Source: CAD feature listing. Evaluate the final solid. Frame: model axes, mm. A direction names the side the tool comes from. Give positions to 0.01 mm unless a question says otherwise; leave off trailing zeros. Order: outer loops, then holes, each group sorted by start corner. A loop starts at its lowest first (then second) coordinate and runs counter-clockwise, first axis right, second up. Notation, with made-up numbers: M -22,39.25 L 2,39.25 A27 ccw 2,63.25 Z; hole C -7.5,-10.5 d9. An arc over 180 degrees is marked long. Answer as a JSON object with one key per item and string values. Group by question number.
1. Section query D-D (x = -15). Output: boundary loops of the cut face in (y, z), plus the area to 3 significant figures.
2. Pin query (flat end, axial travel): P1, Ø8, axis at x = -4, z = 11, coming from the -Y side; P2, Ø3.5, axis at y = -14.5, z = 22, coming from the -X side; P3, Ø8, axis at x = 30, z = -2.5, coming from the -Y side; P4, Ø8, axis at x = 24, y = -16, coming from the +Z side. Return the tip coordinate at first contact, or that it passes through.
3. Material intervals for L1, parallel to Y at x = -6, z = -1; L2, parallel to Y at x = 11, z = 0; L3, parallel to X at y = -17, z = -20, sorted ascending. Write a range as [from, to].
4. Pull-direction query (X, two-part tool) for faces 1 (the flat face through (13.344, -9, 20)), 2 (the flat face through (38.832, 9.524, 16.58)), 3 (the flat face through (16, -6, -14.07)); classes: +X half, -X half, draft (parallel to the pull), parting line (faces both ways), or undercut.
5. Set-up query: faces 4 (the flat face through (16, -6, 14.099)), 5 (the flat face through (13.344, -9, -20)), 6 (the flat face through (38.832, 9.524, -16.342)), 7 (the flat face through (38.45, 12.22, -16.34)). Return all of +Z, -Z, +X, -X, +Y, -Y with unobstructed straight access to the full face (end or side cutting, diameter ignored); none if empty.
6. Section query B-B (x = 16.5). Output: boundary loops of the cut face in (y, z).
7. Section query A-A (y = -3.5). Output: boundary loops of the cut face in (x, z), plus the area to 3 significant figures.
8. Section query C-C (y = -9). Output: boundary loops of the cut face in (x, z), plus the area to 3 significant figures.
from build123d import *

# Parameters (mm, degrees)
F1_DEPTH      = 25.4
F1_DEPTH_BACK = 25.4
F2_W          = 5.8462059447
F2_H          = 15.0438407436
F3_DEPTH      = 2.1542214913
F4_W          = 23.189639207
F4_H          = 28.1684854999
F5_DEPTH      = 8.088287329


with BuildPart() as f1:
    # F0 (on Top) → F1 (new body, two sides)
    with BuildSketch(Plane.XY) as f1_sk:
        with BuildLine():
            Line((39.8870706558, 9.2431334779), (42.8255088627, 20.2876105905))
            Line((42.8255088627, 20.2876105905), (-42.8958497941, 20.2876105905))
            Line((-42.8958497941, 20.2876105905), (-43.1476103375, 19.3413379916))
            Line((-43.1476103375, 19.3413379916), (4.8284521326, 12.586873956))
            add(Edge.make_bspline(
                [(4.8284521326, 12.586873956), (8.3748446777, 11.9789214805), (13.0701588605, 9.1844080016), (13.3440204307, 2.9022279195)],
                knots=[0, 0, 0, 0, 12.8960176912, 12.8960176912, 12.8960176912, 12.8960176912], degree=3))
            Line((13.3440204307, 2.9022279195), (13.3440204307, -20.2874112874))
            Line((13.3440204307, -20.2874112874), (15.2615886182, -20.2874112874))
            Line((15.2615886182, -20.2874112874), (25.4958156311, 18.1791747184))
            Line((25.4958156311, 18.1791747184), (39.0742355021, 14.5665684056))
            Line((39.0742355021, 14.5665684056), (37.8052698946, 9.7970069509))
            Line((37.8052698946, 9.7970069509), (39.8870706558, 9.2431334779))
        make_face()
    extrude(amount=F1_DEPTH)
    extrude(f1_sk.sketch, amount=-F1_DEPTH_BACK)

    # F2 (on face) → F3 (cut, through all)
    with BuildSketch(Plane(origin=(34.9536834808, -9.2996017797, 0), x_dir=(0.2571107359, 0.966381948, 0), z_dir=(0.966381948, -0.2571107359, 0))):
        with Locations((22.1108943995, -0.0125817023)):
            Rectangle(F2_W, F2_H)
    extrude(amount=-F3_DEPTH, mode=Mode.SUBTRACT)

    # F4 (on face) → F5 (cut, through all)
    with BuildSketch(Plane(origin=(13.3440204307, 0, 0), x_dir=(0, -1, 0), z_dir=(-1, 0, 0))):
        with Locations((8.6925916839, 0.0144629739)):
            Rectangle(F4_W, F4_H)
    extrude(amount=-F5_DEPTH, mode=Mode.SUBTRACT)


solid = f1.part
Answer sheet:
{
 "1": {"outline": "M 15.38,-25.4 L 20.29,-25.4 L 20.29,25.4 L 15.38,25.4 Z", "area": "249 mm^2"},
 "2": {"P1": "y = 13.27", "P2": "x = 13.34", "P3": "y = 15.92", "P4": "through"},
 "3": {"L1": "[14.11, 20.29]", "L2": "[9.15, 20.29]", "L3": "[13.34, 16.14]"},
 "4": {"face 1": "-X half", "face 2": "undercut", "face 3": "draft"},
 "5": {"face 4": "+X, -X, -Y", "face 5": "+Z, -Z, -X, -Y", "face 6": "+Z, -Z, -Y", "face 7": "+Z, -Z"},
 "6": {"outline": "M -15.63,-25.4 L 20.29,-25.4 L 20.29,25.4 L -15.63,25.4 L -15.63,14.1 L 2.9,14.1 L 2.9,-14.07 L -15.63,-14.07 Z"},
 "7": {"outline": "M 13.34,-25.4 L 19.73,-25.4 L 19.73,-14.07 L 13.34,-14.07 Z; M 13.34,14.1 L 19.73,14.1 L 19.73,25.4 L 13.34,25.4 Z", "area": "144 mm^2"},
 "8": {"outline": "M 13.34,-25.4 L 18.26,-25.4 L 18.26,-14.07 L 13.34,-14.07 Z; M 13.34,14.1 L 18.26,14.1 L 18.26,25.4 L 13.34,25.4 Z", "area": "111 mm^2"}
}
